Autodesk Inventor part; units mm, degrees
ref_plane "YZ Plane" through (0, 0, 0) normal (1, 0, 0) x (0, 1, 0)
ref_plane "XZ Plane" through (0, 0, 0) normal (0, 1, 0) x (-1, 0, 0)
ref_plane "XY Plane" through (0, 0, 0) normal (0, 0, 1) x (1, 0, 0)
sketch "main" plane through (0, 0, 0) normal (0, 0, 1) x (1, 0, 0)
  line L0 (-27.3481, 7.6574) -> (-27.3481, 8.0441)
  circle A0 centre (-20.9981, -17.7426) radius 2.0955
  line L1 (-27.3481, -43.1426) -> (-27.3481, 8.0441)
  line L2 (-16.7649, -47.8757) -> (-3.0065, -35.5705)
  circle A1 centre (-20.9981, -43.1426) radius 2.0955
  arc A2 (-27.3481, -43.1426) -> (-20.9981, -49.4926) centre (-20.9981, -43.1426) ccw
  arc A3 (-27.3481, -43.1426) -> (-16.7649, -47.8757) centre (-20.9981, -43.1426) ccw
  arc A4 (21.4453, 45.7574) -> (15.0953, 52.1074) centre (15.0953, 45.7574) ccw
  arc A5 (-18.881, 26.9766) -> (-27.3481, 8.0441) centre (-1.9481, 8.0441) ccw
  line L3 (21.4453, 45.7574) -> (21.4453, -5.0426)
  line L4 (5.602, 48.8737) -> (-18.881, 26.9766)
  circle A6 centre (15.0953, 45.7574) radius 2.1844
  line L5 (15.0953, 52.1074) -> (14.0684, 52.1074)
  arc A7 (14.0684, 52.1074) -> (5.602, 48.8737) centre (14.0684, 39.4074) ccw
  circle A8 centre (15.0953, -5.0426) radius 2.1844
  arc A9 (15.0953, -11.3926) -> (21.4453, -5.0426) centre (15.0953, -5.0426) ccw
  line L6 (15.0953, -11.3926) -> (1.2269, -11.3926)
  line L7 (-1.9481, -14.5676) -> (-1.9481, -33.2039)
  arc A10 (1.2269, -11.3926) -> (-1.9481, -14.5676) centre (1.2269, -14.5676) ccw
  arc A11 (-3.0065, -35.5705) -> (-1.9481, -33.2039) centre (-5.1231, -33.2039) ccw
  point P0 (-2.0277, 1.4023)
  point P1 (-1.9481, -34.6239)
  point P2 (9.2176, 52.1074)
  dimension "d1" = 12.7
  dimension "d5" = 4.191
  dimension "d6" = 4.191
  dimension "d8" = 4.3688
  dimension "d9" = 3.175
  dimension "d10" = 25.4
sketch "Sketch1" plane through (0, 0, 0) normal (0, 0, 1) x (1, 0, 0)
  circle A0 centre (-36.0934, -76.2) radius 2.0955
  line L0 (-42.4434, -38.1) -> (-42.4434, -37.7133)
  circle A1 centre (-36.0934, -63.5) radius 2.0955
  line L1 (-42.4434, -88.9) -> (-42.4434, -37.7133)
  line L2 (-31.8602, -93.6331) -> (-18.1018, -81.3279)
  circle A2 centre (-36.0934, -88.9) radius 2.0955
  arc A3 (-42.4434, -88.9) -> (-36.0934, -95.25) centre (-36.0934, -88.9) ccw
  arc A4 (-42.4434, -88.9) -> (-31.8602, -93.6331) centre (-36.0934, -88.9) ccw
  arc A5 (6.35, 0) -> (0, 6.35) centre (0, 0) ccw
  arc A6 (-33.9762, -18.7808) -> (-42.4434, -37.7133) centre (-17.0434, -37.7133) ccw
  line L3 (6.35, 0) -> (6.35, -50.8)
  line L4 (-9.4933, 3.1162) -> (-33.9762, -18.7808)
  circle A7 centre (0, 0) radius 2.1844
  line L5 (0, 6.35) -> (-1.0269, 6.35)
  arc A8 (-1.0269, 6.35) -> (-9.4933, 3.1162) centre (-1.0269, -6.35) ccw
  circle A9 centre (0, -50.8) radius 2.1844
  arc A10 (0, -57.15) -> (6.35, -50.8) centre (0, -50.8) ccw
  line L6 (0, -57.15) -> (-13.8684, -57.15)
  line L7 (-17.0434, -60.325) -> (-17.0434, -78.9613)
  arc A11 (-13.8684, -57.15) -> (-17.0434, -60.325) centre (-13.8684, -60.325) ccw
  arc A12 (-18.1018, -81.3279) -> (-17.0434, -78.9613) centre (-20.2184, -78.9613) ccw
  point P0 (-42.4434, -38.1)
  dimension "d4" = 4.191
extrude "Extrusion1" add sketch "Sketch1" along normal blind 1.5875
properties part number "sled" material "Acetal Resin, White"
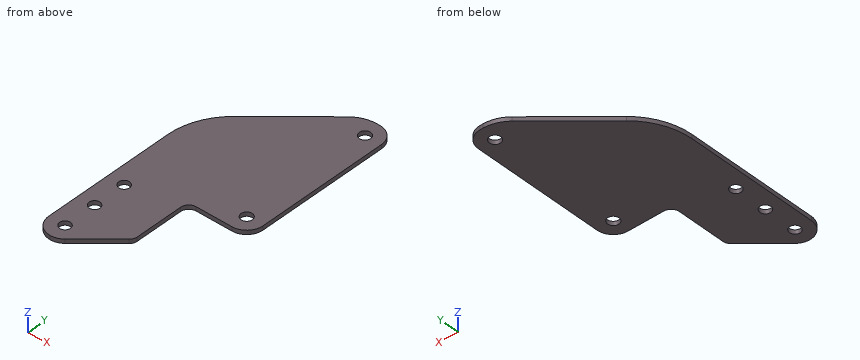
CAD build for the part. Positions are in the model's coordinates, mm. Round coordinates to 2 decimals unless told otherwise and drop trailing zeros. Loops run counter-clockwise (first coordinate to the right, second up) from the corner with the lowest first, then second, coordinate; pieces in that order, holes last.
(1) Cut at D-D (y = -14.5). Give the cut face in (x, z).
(2) Wall check: line 1 along Y through (x, z) = (0, 1.2); line 2 along Y through (x, z) = (-36.5, 0.2); line 3 along X through (y, z) = (-70, 0.75). Give the ranges that are in metal, low to high.
(3) Cut at A-A (y = -76.2). Give the cut face in (x, z), plus the area to 3 significant figures.
(4) Drop flat-ended pins along their axis: pin 1 (0.8 mm diameter, centred on y = -72.5, z = 1, fed in from +X); pin 2 (0.5 mm diameter, centred on x = -7, z = 0.5, fed in from -Y). Give the stop position or say it passes through.
(5) Cut at C-C (x = -15). Give the cut face in (y, z), plus the area to 3 significant figures.
(6) Cut at B-B (z = 0.8). State how many separate pieces and enclosed holes the cut face has, plus the area to 3 significant figures.
Findings below:
1. outline: (-29.19, 0) - (6.35, 0) - (6.35, 1.59) - (-29.19, 1.59) - close
2. line 1: y = -57.15 to -52.98, -48.62 to -2.18, 2.18 to 6.35
2. line 2: y = -95.24 to -90.96, -86.84 to -78.26, -74.14 to -65.56, -61.44 to -21.39
2. line 3: x = -42.44 to -17.04
3. outline: (-42.44, 0) - (-38.19, 0) - (-38.19, 1.59) - (-42.44, 1.59) - close; (-34, 0) - (-17.04, 0) - (-17.04, 1.59) - (-34, 1.59) - close
3. area: 33.7 mm2
4. pin 1: stops at x = -17.04
4. pin 2: stops at y = -57.15
5. outline: (-57.36, 0) - (-1.81, 0) - (-1.81, 1.59) - (-57.36, 1.59) - close
5. area: 88.2 mm2
6. separate pieces: 1
6. enclosed holes: 5
6. area: 3,230 mm2
